Input: part model. Units: mm. Frame: model coordinates. Face numbers are marked on the shaded views. A direction names the side the tool comes from. Coordinates: 2 decimals unless noted, no trailing zeros. Order: outer loops, then holes, each group sorted by start corner. A loop starts at its lowest first (then second) coordinate and runs counter-clockwise, first axis right, second up. Notation, with made-up numbers: M 89,-29 L 142,-29 A18 cw 142,-22 Z; hole C 62,74.5 d5. An arc over 180 degrees is marked long. One line per item, written item: value.
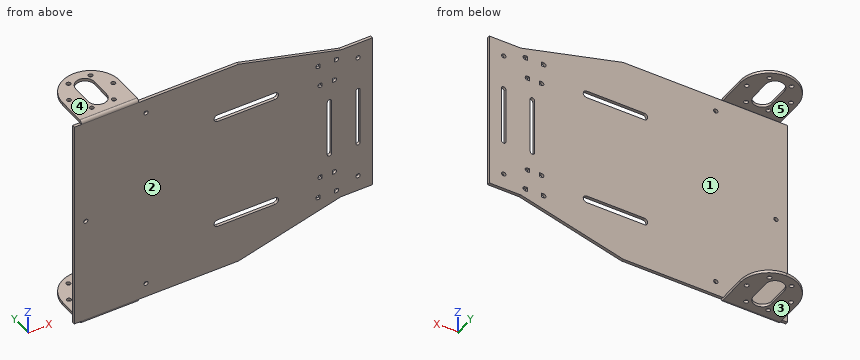
```python
from build123d import *

# Parameters (mm, degrees)
BRIDA_BASE1_DEPTH           = 2
CROQUIS5_R                  = 1.5
CORTAR_EXTRUIR1_DEPTH       = 10
PLIEGUE_START               = -123.687
PLIEGUE_CROQUIZADO1_DEPTH   = 40
PLIEGUE_CROQUIZADO1_2_DEPTH = 40
CROQUIS7_R                  = 1.5
CORTAR_EXTRUIR2_DEPTH       = 206.264173359


# Read off the part's stored shape, not the designer's step: Pliegue croquizado1
# Sheet-metal steps are written as plain solids
with BuildPart() as part:
    # Croquis base → Brida base1 (new body)
    with BuildSketch(Plane(origin=(0, 0, 0), x_dir=(1, 0, 0), z_dir=(0, 1, 0))):
        Polygon((-14.061, -75), (-83.687, -75), (-83.687, -119), (-123.687, -119), (-123.687, -75), (-128.687, -75), (-128.687, 75), (-123.687, 75), (-123.687, 119), (-83.687, 119), (-83.687, 75), (-14.061, 75), (57.313, 56), (79.313, 56), (79.313, -56), (57.313, -56), align=None)
    extrude(amount=-BRIDA_BASE1_DEPTH)

    # Croquis5 → Cortar-Extruir1 (cut)
    with BuildSketch(Plane(origin=(0, 0, 0), x_dir=(1, 0, 0), z_dir=(0, 1, 0))):
        with Locations(Location((-78.687, -65, 0), (0, 0, 270))):
            Circle(CROQUIS5_R)
        with Locations(Location((69.313, -45, 0), (0, 0, 270))):
            Circle(CROQUIS5_R)
        with Locations(Location((69.313, 45, 0), (0, 0, 90))):
            Circle(CROQUIS5_R)
        with Locations(Location((-78.687, 65, 0), (0, 0, 90))):
            Circle(CROQUIS5_R)
        with Locations(Location((-120.687, 0, 0), (0, 0, 270))):
            Circle(CROQUIS5_R)
        with BuildLine():
            Line((-28.687, -37.5), (11.313, -37.5))
            ThreePointArc((11.313, -37.5), (13.813, -40), (11.313, -42.5))
            Line((11.313, -42.5), (-28.687, -42.5))
            ThreePointArc((-28.687, -42.5), (-31.187, -40), (-28.687, -37.5))
        make_face()
        with BuildLine():
            Line((41.313, -51.5), (42.813, -51.5))
            Line((42.813, -51.5), (42.813, -48.5))
            Line((42.813, -48.5), (41.313, -48.5))
            ThreePointArc((41.313, -48.5), (39.813, -50), (41.313, -51.5))
        make_face()
        with BuildLine():
            Line((51.313, 36.5), (52.813, 36.5))
            ThreePointArc((52.813, 36.5), (54.313, 35), (52.813, 33.5))
            Line((52.813, 33.5), (51.313, 33.5))
            Line((51.313, 33.5), (51.313, 36.5))
        make_face()
        with BuildLine():
            Line((52.813, -48.5), (54.313, -48.5))
            ThreePointArc((54.313, -48.5), (55.813, -50), (54.313, -51.5))
            Line((54.313, -51.5), (52.813, -51.5))
            Line((52.813, -51.5), (52.813, -48.5))
        make_face()
        with BuildLine():
            Line((42.813, -33.5), (44.313, -33.5))
            Line((44.313, -33.5), (44.313, -36.5))
            Line((44.313, -36.5), (42.813, -36.5))
            ThreePointArc((42.813, -36.5), (41.313, -35), (42.813, -33.5))
        make_face()
        with BuildLine():
            Line((51.313, -33.5), (52.813, -33.5))
            ThreePointArc((52.813, -33.5), (54.313, -35), (52.813, -36.5))
            Line((52.813, -36.5), (51.313, -36.5))
            Line((51.313, -36.5), (51.313, -33.5))
        make_face()
        with BuildLine():
            Line((44.313, 33.5), (44.313, 36.5))
            Line((44.313, 36.5), (42.813, 36.5))
            ThreePointArc((42.813, 36.5), (41.313, 35), (42.813, 33.5))
            Line((42.813, 33.5), (44.313, 33.5))
        make_face()
        with BuildLine():
            Line((52.813, 51.5), (54.313, 51.5))
            ThreePointArc((54.313, 51.5), (55.813, 50), (54.313, 48.5))
            Line((54.313, 48.5), (52.813, 48.5))
            Line((52.813, 48.5), (52.813, 51.5))
        make_face()
        with BuildLine():
            Line((42.813, 51.5), (42.813, 48.5))
            Line((42.813, 48.5), (41.313, 48.5))
            ThreePointArc((41.313, 48.5), (39.813, 50), (41.313, 51.5))
            Line((41.313, 51.5), (42.813, 51.5))
        make_face()
        with BuildLine():
            Line((-28.687, 37.5), (11.313, 37.5))
            ThreePointArc((11.313, 37.5), (13.813, 40), (11.313, 42.5))
            Line((11.313, 42.5), (-28.687, 42.5))
            ThreePointArc((-28.687, 42.5), (-31.187, 40), (-28.687, 37.5))
        make_face()
        with BuildLine():
            Line((47.813, 20), (47.813, -20))
            ThreePointArc((47.813, -20), (49.313, -21.5), (50.813, -20))
            Line((50.813, -20), (50.813, 20))
            ThreePointArc((50.813, 20), (49.313, 21.5), (47.813, 20))
        make_face()
        with BuildLine():
            Line((67.813, 20), (67.813, -20))
            ThreePointArc((67.813, -20), (69.313, -21.5), (70.813, -20))
            Line((70.813, -20), (70.813, 20))
            ThreePointArc((70.813, 20), (69.313, 21.5), (67.813, 20))
        make_face()
    extrude(amount=-CORTAR_EXTRUIR1_DEPTH, mode=Mode.SUBTRACT)

    # Pliegue croquizado1 outline → Pliegue croquizado1 (cut)
    with BuildSketch(Plane.YZ.offset(PLIEGUE_START)):
        with BuildLine():
            ThreePointArc((0, -77.097617696), (-1.419868415, -76.449137674), (-2, -75))
            Line((-2, -75), (-2, -119))
            Line((-2, -119), (0, -119))
            Line((0, -119), (0, -77.097617696))
        make_face()
        with BuildLine():
            Line((-2, 119), (-2, 75))
            ThreePointArc((-2, 75), (-1.419868415, 76.449137674), (0, 77.097617696))
            Line((0, 77.097617696), (0, 119))
            Line((0, 119), (-2, 119))
        make_face()
    extrude(amount=PLIEGUE_CROQUIZADO1_DEPTH, mode=Mode.SUBTRACT)

    # Pliegue croquizado1 2 outline → Pliegue croquizado1 2 (add)
    with BuildSketch(Plane.YZ.offset(PLIEGUE_START)):
        with BuildLine():
            Line((0, -75), (0, -77.097617696))
            ThreePointArc((0, -77.097617696), (0.049985814, -77.09940434), (0.1, -77.1))
            Line((0.1, -77.1), (42.372124041, -77.1))
            Line((42.372124041, -77.1), (42.372124041, -75.1))
            Line((42.372124041, -75.1), (0.1, -75.1))
            ThreePointArc((0.1, -75.1), (0.029289322, -75.070710678), (0, -75))
        make_face()
        with BuildLine():
            ThreePointArc((0.1, 77.1), (0.049985814, 77.09940434), (0, 77.097617696))
            Line((0, 77.097617696), (0, 75))
            ThreePointArc((0, 75), (0.029289322, 75.070710678), (0.1, 75.1))
            Line((0.1, 75.1), (42.372124041, 75.1))
            Line((42.372124041, 75.1), (42.372124041, 77.1))
            Line((42.372124041, 77.1), (0.1, 77.1))
        make_face()
    extrude(amount=PLIEGUE_CROQUIZADO1_2_DEPTH)

    # Croquis7 → Cortar-Extruir2 (cut, through all)
    with BuildSketch(Plane.XY.offset(77.1)):
        with BuildLine():
            Line((-103.687, 39.5), (-103.687, 42.372124041))
            Line((-103.687, 42.372124041), (-123.687, 42.372124041))
            Line((-123.687, 42.372124041), (-123.687, 19.5))
            ThreePointArc((-123.687, 19.5), (-117.829135624, 33.642135624), (-103.687, 39.5))
        make_face()
        with BuildLine():
            Line((-83.687, 42.372124041), (-103.687, 42.372124041))
            Line((-103.687, 42.372124041), (-103.687, 39.5))
            ThreePointArc((-103.687, 39.5), (-89.544864376, 33.642135624), (-83.687, 19.5))
            Line((-83.687, 19.5), (-83.687, 42.372124041))
        make_face()
        with BuildLine():
            Line((-110.187, 26.5), (-110.187, 12.5))
            ThreePointArc((-110.187, 12.5), (-103.687, 6), (-97.187, 12.5))
            Line((-97.187, 12.5), (-97.187, 26.5))
            ThreePointArc((-97.187, 26.5), (-103.687, 33), (-110.187, 26.5))
        make_face()
        with Locations((-119.187, 19.5)):
            Circle(CROQUIS7_R)
        with Locations((-111.437, 32.823393759)):
            Circle(CROQUIS7_R)
        with Locations((-96.02360254, 32.773393759)):
            Circle(CROQUIS7_R)
        with Locations((-88.360205081, 19.4)):
            Circle(CROQUIS7_R)
        with Locations((-96.110205081, 6.076606241)):
            Circle(CROQUIS7_R)
        with Locations((-111.52360254, 6.126606241)):
            Circle(CROQUIS7_R)
    extrude(amount=-CORTAR_EXTRUIR2_DEPTH, mode=Mode.SUBTRACT)


solid = part.part
```
(1) Access query for the marked faces 1 and 2. Directions: +Z, -Z, +X, -X, +Y, -Y. A direction counts if a zero-diameter tool reaches every point of the face in a straight line with its end or side. Return the directions, or none.
Data:
face 1: +X, -X, +Y
face 2: +Z, -Z, +X, -X, -Y
(2) First-contact query: pin 1 (0.8 mm diameter, centred on x = 52, y = -1.5, fed in from +Z); pin 2 (1 mm diameter, centred on x = -16.5, z = 18, fed in from +Y); pin 3 (1 mm diameter, centred on x = 68, y = -1, fed in from -Z); pin 4 (3.5 mm diameter, centred on x = -88.36, y = 19.4, fed in from -Z). Flat tips, straight axial feed; report the tip coordinate or a pass-through.
Data:
pin 1: stops at z = 57.52
pin 2: stops at y = 0
pin 3: stops at z = -56
pin 4: stops at z = -77.1
(3) Cut plane B-B on x = -26. Output: boundary loops of the cut face in (y, z).
Data:
outline: M -2,-75 L 0,-75 L 0,-42.5 L -2,-42.5 Z; M -2,-37.5 L 0,-37.5 L 0,37.5 L -2,37.5 Z; M -2,42.5 L 0,42.5 L 0,75 L -2,75 Z
(4) Cut plane C-C on y = 37. Output: boundary loops of the cut face in (x, z).
Data:
outline: M -113.37,-77.1 L -94,-77.1 L -94,-75.1 L -113.37,-75.1 Z; M -113.37,75.1 L -94,75.1 L -94,77.1 L -113.37,77.1 Z
(5) Draft query along Z for the marked faces 3, 4 and 5. Return one class per face: released by +Z, released by -Z, zero draft, split by the parting line, or undercut.
Data:
face 3: released by -Z
face 4: released by +Z
face 5: undercut
(6) Ray query, line 1 (Y direction, x = -62.5, z = 40); line 2 (X direction, y = -0.55, z = 45); line 3 (Z direction, x = -90, y = 14.5). Return the intervals inside material, ascending. Write a range as from..to.
Data:
line 1: y = -2..0
line 2: x = -128.69..67.81, 70.81..79.31
line 3: z = -77.1..-75.1, 75.1..77.1
(7) Cut plane A-A on z = 40. Output: boundary loops of the cut face in (x, y).
Data:
outline: M -128.69,-2 L -31.19,-2 L -31.19,0 L -128.69,0 Z; M 13.81,-2 L 79.31,-2 L 79.31,0 L 13.81,0 Z
(8) Cut plane D-D on z = -24. Output: boundary loops of the cut face in (x, y), plus the area to 3 significant figures.
Data:
outline: M -128.69,-2 L 79.31,-2 L 79.31,0 L -128.69,0 Z
area: 416 mm2
